The listing builds one solid part. Answer for the finished solid, in the listing's coordinates (mm). Coordinates: 2 decimals unless noted, no trailing zeros. Loops run counter-clockwise (first coordinate to the right, second up) from the corner with the lowest first, then second, coordinate; pieces in that order, holes last. Notation, with made-up numbers: M 35.25,-25.75 L 60.25,-25.75 A31 ccw 60.25,0.25 Z; hole C 17,56.5 d7. An arc over 180 degrees is marked long. Answer in a Markdown table with one row per item. Add a question column.
from build123d import *

# Parameters (mm, degrees)
F1_DEPTH = 3
F2_W     = 20
F2_H     = 3
F3_DEPTH = 3.001


# Not quite as in the source:
# - a feature names something its author has since deleted; it is built from what else it names


with BuildPart() as f1:
    # F0 (on Top) → F1 (new body)
    with BuildSketch(Plane.XY):
        Polygon((-74, 0), (0, 0), (74, 0), (74, 20), (77, 20), (77, 50), (74, 50), (74, 85), (77, 85), (77, 115), (74, 115), (74, 150), (77, 150), (77, 180), (74, 180), (74, 200), (0, 200), (-74, 200), (-74, 180), (-77, 180), (-77, 150), (-74, 150), (-74, 115), (-77, 115), (-77, 85), (-74, 85), (-74, 50), (-77, 50), (-77, 20), (-74, 20), align=None)
    extrude(amount=F1_DEPTH)

    # F2 (on face) → F3 (cut, through all)
    with BuildSketch(Plane.XY.offset(3)):
        with Locations((-44, 1.5)):
            Rectangle(F2_W, F2_H)
        with Locations((44, 1.5)):
            Rectangle(F2_W, F2_H)
        with Locations((0, 1.5)):
            Rectangle(F2_W, F2_H)
        with Locations((-44, 198.5)):
            Rectangle(F2_W, F2_H)
        with Locations((44, 198.5)):
            Rectangle(F2_W, F2_H)
        with Locations((0, 198.5)):
            Rectangle(F2_W, F2_H)
    extrude(amount=-F3_DEPTH, mode=Mode.SUBTRACT)


solid = f1.part
(1) Straight lines are drawn through the part: line 1 (Y direction, x = 49.5, z = 0.3); line 2 (X direction, y = 116, z = 0.6). For each, find the intervals that lie inside material, in ascending order.
(2) A cutting plane is placed at B-B (x = -47). Give the vertices of the cut face in (y, z), plus the area to 3 significant figures.
(3) Each of these flat-tipped pins is pushed along its axis until it touches: pin 1 (1.5 mm diameter, centred on x = 37.5, z = 2.5, fed in from +Y); pin 2 (1.5 mm diameter, centred on x = 76, z = 2, fed in from +Y); pin 3 (1.5 mm diameter, centred on y = 1.5, z = 2, fed in from +X). Where does it stop, or does it pass through?
(4) A cutting plane is placed at A-A (y = 130). Give the vertices of the cut face in (x, z), plus the area to 3 significant figures.
Solved:
| question | item | result |
|---|---|---|
| 1 | line 1 | y = 3 to 197 |
| 1 | line 2 | x = -74 to 74 |
| 2 | outline | M 3,0 L 197,0 L 197,3 L 3,3 Z |
| 2 | area | 582 mm² |
| 3 | pin 1 | stops at y = 197 |
| 3 | pin 2 | stops at y = 180 |
| 3 | pin 3 | stops at x = 74 |
| 4 | outline | M -74,0 L 74,0 L 74,3 L -74,3 Z |
| 4 | area | 444 mm² |
